from build123d import *

# Parameters (mm, degrees)
SKETCH_R      = 30.15
SKETCH_R_2    = 24.15
PAD_DEPTH     = 48
SKETCH001_R   = 24
SKETCH001_R_2 = 9.5
PAD001_DEPTH  = 10
SKETCH002_R   = 24
SKETCH002_R_2 = 9.5
PAD002_DEPTH  = 10


with BuildPart() as part:
    # Sketch → Pad (new body)
    with BuildSketch(Plane.XY):
        Circle(SKETCH_R)
        Circle(SKETCH_R_2, mode=Mode.SUBTRACT)
    extrude(amount=PAD_DEPTH)

    # Sketch001 → Pad001 (join)
    with BuildSketch(Plane.XZ.offset(-5)):
        with Locations((50, 24.15)):
            Circle(SKETCH001_R)
        with Locations((50, 24.15)):
            Circle(SKETCH001_R_2, mode=Mode.SUBTRACT)
    extrude(amount=PAD001_DEPTH)

    # Sketch002 → Pad002 (join)
    with BuildSketch(Plane.YZ.offset(-5)):
        with Locations((50, 24)):
            Circle(SKETCH002_R)
        with Locations((50, 24)):
            Circle(SKETCH002_R_2, mode=Mode.SUBTRACT)
    extrude(amount=PAD002_DEPTH)


solid = part.part
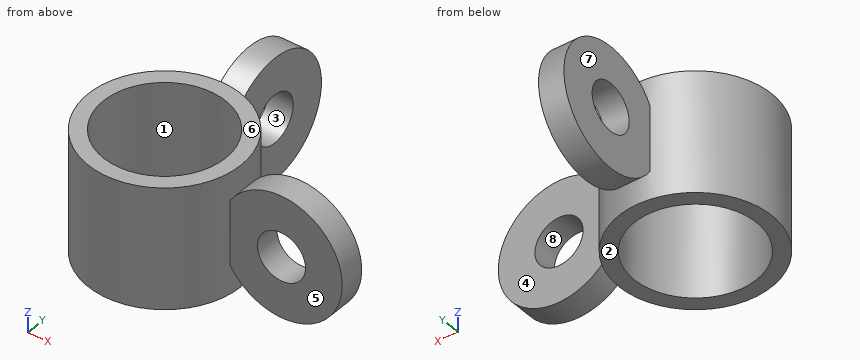
The model under review builds one solid part; all positions refer to its coordinate system, in mm. Face numbers are marked on the shaded views. A direction names the side the tool comes from. Round coordinates to 2 decimals unless told otherwise and drop trailing zeros. Loops run counter-clockwise (first coordinate to the right, second up) from the corner with the lowest first, then second, coordinate; pieces in that order, holes last. Notation, with made-up numbers: M -28.75,50 L 28.25,50 A22 ccw 28.25,82 Z; hole C 40.5,77 d6. An arc over 180 degrees is marked long. Answer as a JSON object with one key per item and string values.
Item 1: We need section C-C, the plane x = 50. State the section outline as (y, z) points.
Check sheet entries:
{"outline": "M -5,0.15 L 5,0.15 L 5,14.65 L -5,14.65 Z; M -5,33.65 L 5,33.65 L 5,48.15 L -5,48.15 Z"}
Item 2: We need section A-A, the plane y = 0. State the section outline as (x, z) points.
Check sheet entries:
{"outline": "M -30.15,0 L -24.15,0 L -24.15,48 L -30.15,48 Z; M 24.15,0 L 30.15,0 L 30.15,10.66 A24 ccw long 30.15,37.64 L 30.15,48 L 24.15,48 Z; hole C 50,24.15 d19"}
Item 3: For line 1 along Z through (x, y) = (50, 3); line 2 along Z through (x, y) = (16.5, -19.5); line 3 along X through (y, z) = (-10, 15), list the stretches that pass through material, from the lowest coordinate up.
Check sheet entries:
{"line 1": "0.15 to 14.65, 33.65 to 48.15", "line 2": "0 to 48", "line 3": "-28.44 to -21.98, 21.98 to 28.44"}
Item 4: Clearance check with flat-ended pins moving along their axes: P1, Ø2, axis at y = 8, z = 10, coming from the -X side; P2, Ø1, axis at x = 18, z = 14, coming from the +Y side; P3, Ø4, axis at x = 22, z = 15, coming from the -Y side. State where each tip first meets the part, or that it passes through.
Check sheet entries:
{"P1": "x = -29.33", "P2": "y = 24.55", "P3": "y = -22.56"}
Item 5: We need section B-B, the plane x = 0. State the section outline as (y, z) points, and give its area (3 significant figures).
Check sheet entries:
{"outline": "M -30.15,0 L -24.15,0 L -24.15,48 L -30.15,48 Z; M 24.15,0 L 30.15,0 L 30.15,10.51 A24 ccw long 30.15,37.49 L 30.15,48 L 24.15,48 Z; hole C 50,24 d19", "area": "2,030 mm2"}
Item 6: We need section D-D, the plane z = 8. State the section outline as (x, y) points, and give its area (3 significant figures).
Check sheet entries:
{"outline": "C 0,0 d60.3; M -5,32.11 L 5,32.11 L 5,67.89 L -5,67.89 Z; M 32.25,-5 L 67.75,-5 L 67.75,5 L 32.25,5 Z; hole C 0,0 d48.3", "area": "1,740 mm2"}
Item 7: The part is to be moulded in two halves that separate along Z. For the marked faces 1, 2 and 3, say which applies: +Z half, -Z half, draft (parallel to the pull), parting line (faces both ways), or undercut.
Check sheet entries:
{"face 1": "draft", "face 2": "-Z half", "face 3": "undercut"}
Item 8: Tool access review of the marked faces 4, 5, 6, 7 and 8: name each direction out of +Z, -Z, +X, -X, +Y, -Y from which nothing blocks a thin tool from reaching the whole face with its end or side.
Check sheet entries:
{"face 4": "+Z, -Z, +X, +Y", "face 5": "+Z, -Z, +X, -Y", "face 6": "+Z, -X, +Y, -Y", "face 7": "+Z, -Z, -X, +Y", "face 8": "+Y, -Y"}
